Read the model definition and answer for the solid it produces. Units are mm, in the model's axes. A direction names the side the tool comes from. Give positions to 0.01 mm unless a question says otherwise; leave off trailing zeros. Loops run counter-clockwise (first coordinate to the right, second up) from the corner with the lowest first, then second, coordinate; pieces in that order, holes last. Notation, with made-up numbers: (7.5, -4) - (49.5, -4) arc R27 ccw to (49.5, 21) - close; hole circle Ø6 at (35.25, 26). An arc over 180 degrees is marked (long way). Put each result on its own line as item: value. Start each with the question number.
1. For a pull along Y with two mould halves and no side action, classify faces 1 (the flat face through (-10, -45.589, 3)), 2 (the flat face through (0, -35, 0)), 3 (the flat face through (-32, -28.3, 13)), 4 (the flat face through (31, -38.91, 13)) as released by +Y, released by -Y, zero draft, split by the parting line, or undercut.
2. A cutting plane is placed at A-A, the plane z = 12. Determine the outline of the cut face in (x, y).
3. A cutting plane is placed at C-C, the plane y = -16.5. Determine the outline of the cut face in (x, z).
4. For faces 5 (the flat face through (-18.353, -34, 13)), 6 (the flat face through (20.074, -75, 3)), 7 (the flat face through (0, 33, 2)), 8 (the flat face through (-9.048, 15, 2)), determine the directions among +Z, -Z, +X, -X, +Y, -Y from which every point of the face is accessible in a straight line to the end or side of a thin tool.
5. Consider L1, parallel to Y at x = -32, z = 3.75; L2, parallel to Y at x = 20.5, z = 4.75; L3, parallel to Y at x = 2, z = 3.25. Determine where each line is inside the solid, lowest interval first. Write a range as from..to.
6. A cutting plane is placed at B-B, the plane x = -23.5. Determine the outline of the cut face in (y, z), plus the area to 3 significant figures.
7. A cutting plane is placed at D-D, the plane x = -4. Determine the outline of the cut face in (y, z), plus the area to 3 significant figures.
8. Given pin 1 Ø4 at (y, z) = (13.5, 1.5) entering from -X; pin 2 Ø10 at (x, y) = (9, -41) entering from +Z; pin 3 Ø5 at (x, z) = (-26.5, 16.5) entering from +Y, each flat-ended and moving along its own axis, determine where each tip first touches the part or whether it passes through.
```python
from build123d import *

# Parameters (mm, degrees)
BASE_DEPTH                = 5
ESBO_O2_W                 = 71.017341725
ESBO_O2_H                 = 15.188699459
SENSOR_DEPTH              = 3
EXTENS_O_BASE_BY          = 41.124942484
ESBO_O3_W                 = 68.089828176
ESBO_O3_H                 = 2.204794608
FURO_SENSOR_DEPTH         = 10
ESBO_O5_R                 = 1.188185025
ESBO_O5_R_2               = 1.258078261
ESBO_O5_R_3               = 1.220632904
CONECTOR_RODA_BAMBA_DEPTH = 10
ESBO_O8_W                 = 20.37740853
ESBO_O8_H                 = 20.377408531
PONTE_H_DEPTH             = 2
ESBO_O10_W                = 57.764058892
ESBO_O10_H                = 27.282150264
ESP_DEPTH                 = 2
ESBO_O11_W                = 27.929189737
ESBO_O11_H                = 10.609725103
ESBO_O11_W_2              = 26.320868842
RESSALTO_EXTRUS_O2_DEPTH  = 16
ESBO_O13_W                = 60.293581274
ESBO_O13_H                = 57.562513133
CORTE_EXTRUS_O12_DEPTH    = 4


with BuildPart() as part:
    # Esboço1 → base (new body)
    with BuildSketch(Plane.XY):
        Polygon((-44.67348187, 40.715072084), (-44.67348187, 19.603553226), (-9.047793796, 19.603553226), (-9.047793796, 9.424785205), (-44.67348187, 9.424785205), (-44.67348187, -71.439871851), (45.61596039, -71.439871851), (45.61596039, 9.424785205), (10.178768021, 9.424785205), (10.178768021, 19.603553226), (45.61596039, 19.603553226), (45.61596039, 40.715072084), align=None)
    extrude(amount=BASE_DEPTH)

    # Esboço2 → sensor (cut)
    with BuildSketch(Plane.XY.offset(5)):
        with Locations((0.47123926, 33.120722355)):
            Rectangle(ESBO_O2_W, ESBO_O2_H)
    extrude(amount=-SENSOR_DEPTH, mode=Mode.SUBTRACT)

    # extensão base: a face moved outward by 41.124942
    extrude(part.faces().sort_by_distance((0.47123926, -71.439871851, 2.5))[0], amount=EXTENS_O_BASE_BY, dir=(0, -1, 0))

    # Esboço3 → "furo" sensor (cut)
    with BuildSketch(Plane.XY.offset(2)):
        with Locations((0.67810757, 38.709026673)):
            Rectangle(ESBO_O3_W, ESBO_O3_H)
    extrude(amount=-FURO_SENSOR_DEPTH, mode=Mode.SUBTRACT)

    # Esboço5 → conector roda bamba (cut)
    with BuildSketch(Plane(origin=(0, 0, 0), x_dir=(-1, 0, 0), z_dir=(0, 0, -1))):
        with Locations((-8.517583176, -50.2919249)):
            Circle(ESBO_O5_R)
        with Locations((-8.517583176, -64.550145197)):
            Circle(ESBO_O5_R_2)
        with Locations((8.885832774, -64.550145197)):
            Circle(ESBO_O5_R_3)
        with Locations((8.885832774, -50.2919249)):
            Circle(ESBO_O5_R)
    extrude(amount=-CONECTOR_RODA_BAMBA_DEPTH, mode=Mode.SUBTRACT)

    # Esboço8 → ponte H (cut)
    with BuildSketch(Plane.XY.offset(5)):
        with Locations((-31.939333104, -4.30205468)):
            Rectangle(ESBO_O8_W, ESBO_O8_H)
    extrude(amount=-PONTE_H_DEPTH, mode=Mode.SUBTRACT)

    # Esboço10 → esp (cut)
    with BuildSketch(Plane.XY.offset(5)):
        with Locations((12.550316437, -8.596467221)):
            Rectangle(ESBO_O10_W, ESBO_O10_H)
    extrude(amount=-ESP_DEPTH, mode=Mode.SUBTRACT)

    # Esboço11 → Ressalto-extrusão2 (add)
    with BuildSketch(Plane.XY.offset(5)):
        with Locations((31.651365522, -33.605104963)):
            Rectangle(ESBO_O11_W, ESBO_O11_H)
        with Locations((-31.513047449, -33.605104963)):
            Rectangle(ESBO_O11_W_2, ESBO_O11_H)
    extrude(amount=RESSALTO_EXTRUS_O2_DEPTH)

    # Esboço13 → Corte-extrusão12 (cut)
    with BuildSketch(Plane.XY.offset(5)):
        with Locations((-10.073047237, -74.36990727)):
            Rectangle(ESBO_O13_W, ESBO_O13_H)
    extrude(amount=-CORTE_EXTRUS_O12_DEPTH, mode=Mode.SUBTRACT)


solid = part.part
```
Return value:
1. face 1: undercut
1. face 2: zero draft
1. face 3: released by +Y
1. face 4: released by -Y
2. outline: (-44.67, -38.91) - (-18.35, -38.91) - (-18.35, -28.3) - (-44.67, -28.3) - close; (17.69, -38.91) - (45.62, -38.91) - (45.62, -28.3) - (17.69, -28.3) - close
3. outline: (-44.67, 0) - (45.62, 0) - (45.62, 5) - (41.43, 5) - (41.43, 3) - (-16.33, 3) - (-16.33, 5) - (-44.67, 5) - close
4. face 5: +Z, +Y, -Y
4. face 6: +Z
4. face 7: +Z, +Y
4. face 8: +Z, -Z, -X
5. L1: y = -112.56..-103.15, -45.59..-14.49, 5.89..9.42, 19.6..25.53
5. L2: y = -112.56..-22.24, 5.04..9.42, 19.6..25.53
5. L3: y = -112.56..-103.15, -45.59..-22.24, 5.04..25.53
6. outline: (-112.56, 0) - (9.42, 0) - (9.42, 5) - (5.89, 5) - (5.89, 3) - (-14.49, 3) - (-14.49, 5) - (-28.3, 5) - (-28.3, 21) - (-38.91, 21) - (-38.91, 5) - (-45.59, 5) - (-45.59, 1) - (-103.15, 1) - (-103.15, 5) - (-112.56, 5) - close; (19.6, 0) - (37.61, 0) - (37.61, 2) - (25.53, 2) - (25.53, 5) - (19.6, 5) - close; (39.81, 0) - (40.72, 0) - (40.72, 2) - (39.81, 2) - close
6. area: 564 mm2
7. outline: (-112.56, 0) - (37.61, 0) - (37.61, 2) - (25.53, 2) - (25.53, 5) - (5.04, 5) - (5.04, 3) - (-22.24, 3) - (-22.24, 5) - (-45.59, 5) - (-45.59, 1) - (-103.15, 1) - (-103.15, 5) - (-112.56, 5) - close; (39.81, 0) - (40.72, 0) - (40.72, 2) - (39.81, 2) - close
7. area: 432 mm2
8. pin 1: stops at x = -9.05
8. pin 2: stops at z = 5
8. pin 3: stops at y = -28.3
